Answer from the drawing. Dimensions are ordinates in mm from the lowest x, y and z of the part. Round coordinates to 2 decimals unless told otherwise and drop trailing zeros. Loops run counter-clockwise (first coordinate to the right, second up) from the corner with the lowest first, then second, coordinate; pieces in that order, holes last. Notation, with made-up numbers: M 24,85 L 43,85 A5 cw 43,92 Z; hole C -25.75,49.5 d9. An arc over 180 degrees is marked long. Write each question's results on one line, items separated by ' | '.
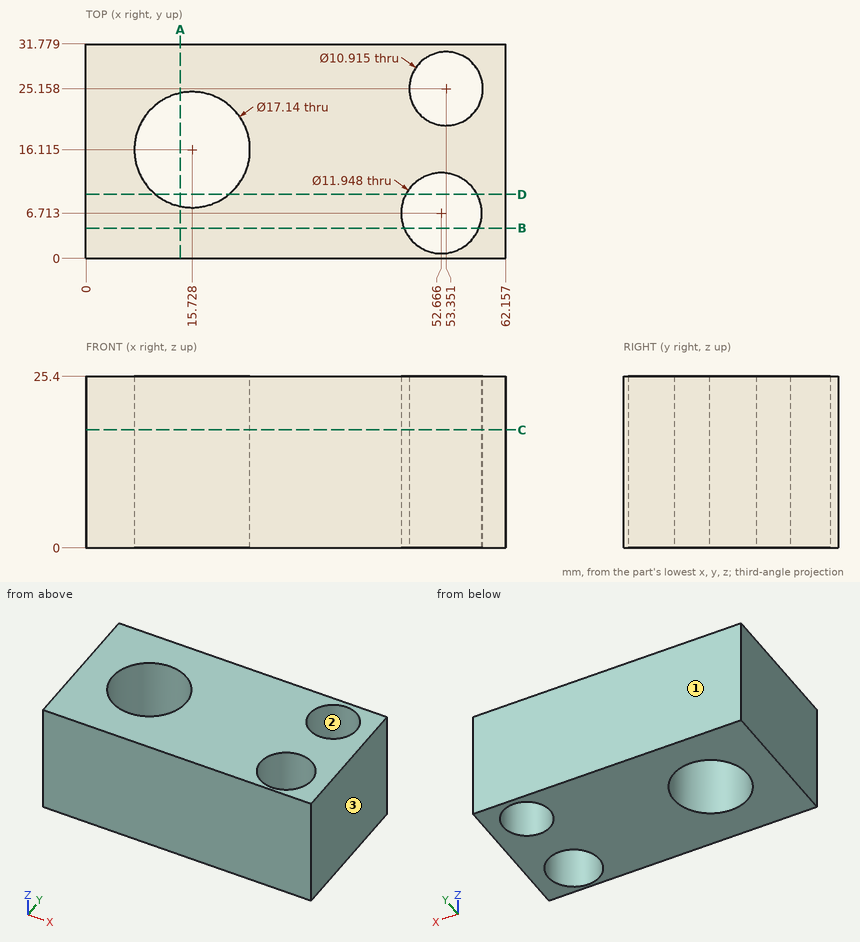
1. Determine the mould class of the marked faces 1, 2 and 3 for opening direction Y: released by +Y, released by -Y, zero draft, split by the parting line, or undercut.
Completed:
face 1: released by +Y | face 2: undercut | face 3: zero draft
2. Find the intervals of material crossed by L1, parallel to Y at x = 53.5, z = 24.25; L2, parallel to X at y = 20.5, z = 22 (1 decimal); L3, parallel to Y at x = 57.5, z = 3 (1 decimal), in increasing order.
Completed:
L1: y = 0 to 0.8, 12.63 to 19.7, 30.61 to 31.78 | L2: x = 0 to 8.4, 23.1 to 50.5, 56.2 to 62.2 | L3: y = 0 to 3.2, 10.2 to 21.6, 28.7 to 31.8
3. Find section D-D, the plane y = 9.5. Give the vertices of the cut face in (x, z).
Completed:
outline: M 0,0 L 10.28,0 L 10.28,25.4 L 0,25.4 Z; M 21.18,0 L 47.38,0 L 47.38,25.4 L 21.18,25.4 Z; M 57.95,0 L 62.16,0 L 62.16,25.4 L 57.95,25.4 Z
4. Find section A-A, the plane x = 14. Give the vertices of the cut face in (y, z).
Completed:
outline: M 0,0 L 7.72,0 L 7.72,25.4 L 0,25.4 Z; M 24.51,0 L 31.78,0 L 31.78,25.4 L 24.51,25.4 Z
5. Find section C-C, the plane z = 17.5. Count the separate pieces of the cut face and the enclosed holes in it, then the cut area to 3 significant figures.
Completed:
separate pieces: 1 | enclosed holes: 3 | area: 1,540 mm2
6. Find section B-B, the plane y = 4.5. Give the vertices of the cut face in (x, z) (1 decimal).
Completed:
outline: M 0,0 L 47.1,0 L 47.1,25.4 L 0,25.4 Z; M 58.2,0 L 62.2,0 L 62.2,25.4 L 58.2,25.4 Z
